The listing builds one solid part. Answer for the finished solid, in the listing's coordinates (mm). Face numbers are marked on the shaded views. A direction names the side the tool comes from. Coordinates: 2 decimals unless noted, no trailing zeros. Write each loop counter-clockwise with the first axis right and the second up, starting at its lowest first coordinate (ties: lowest second). Pieces come first, ordered by that corner, then holes.
(1) The part is cut by section A-A on x = 20. Determine the outline of the cut face in (y, z), plus the area to 3 significant figures.
(2) The part is cut by section C-C on y = 11. Determine the outline of the cut face in (x, z).
(3) Straight lines are drawn through the part: line 1 (Y direction, x = 20, z = 2.5); line 2 (X direction, y = 23.5, z = 14); line 3 (Z direction, x = 264, y = 31). For each, find the intervals that lie inside material, in ascending order.
(4) The part is cut by section B-B on z = 4.5. Determine the outline of the cut face in (x, y).
(5) Which of the six approach directions +Z, -Z, +X, -X, +Y, -Y give full straight-line access (tool end or side, diameter ignored) to the marked faces 1, 2 and 3?
(6) Given P1, Ø5, axis at y = 18.5, z = 14, coming from the -X side; P2, Ø20, axis at x = 19, y = 28.5, coming from the +Z side; P3, Ø11, axis at y = 14, z = 17.5, coming from the +X side, each flat-ended and moving along its own axis, determine where each tip first touches the part or whether it passes through.
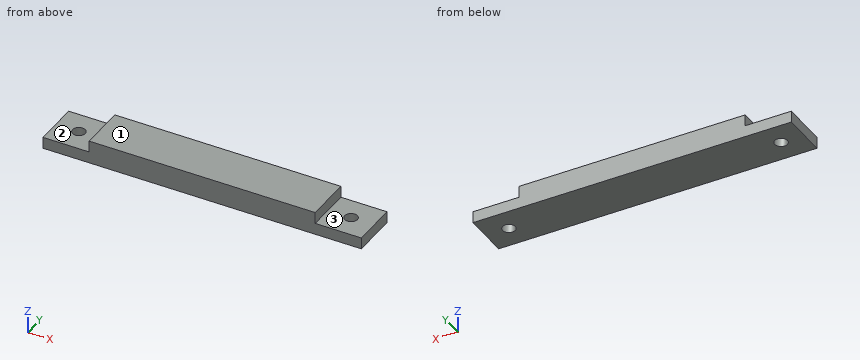
from build123d import *

# Parameters (mm, degrees)
ESQUISSE1_W        = 275.97
ESQUISSE1_H        = 40
ESQUISSE1_R        = 5.5
BOSS_EXTRU_1_DEPTH = 10
ESQUISSE2_W        = 195.97
ESQUISSE2_H        = 40
BOSS_EXTRU_2_DEPTH = 10


with BuildPart() as part:
    # Esquisse1 → Boss.-Extru.1 (new body)
    with BuildSketch(Plane.XY):
        with Locations((137.985, 20)):
            Rectangle(ESQUISSE1_W, ESQUISSE1_H)
        with Locations((20, 20)):
            Circle(ESQUISSE1_R, mode=Mode.SUBTRACT)
        with Locations(Location((255.97, 20, 0), (0, 0, 180))):
            Circle(ESQUISSE1_R, mode=Mode.SUBTRACT)
    extrude(amount=BOSS_EXTRU_1_DEPTH)

    # Esquisse2 → Boss.-Extru.2 (add)
    with BuildSketch(Plane.XY.offset(10)):
        with Locations((137.985, 20)):
            Rectangle(ESQUISSE2_W, ESQUISSE2_H)
    extrude(amount=BOSS_EXTRU_2_DEPTH)


solid = part.part
Model answer:
1. outline: (0, 0) - (14.5, 0) - (14.5, 10) - (0, 10) - close; (25.5, 0) - (40, 0) - (40, 10) - (25.5, 10) - close
1. area: 290 mm2
2. outline: (0, 0) - (275.97, 0) - (275.97, 10) - (235.97, 10) - (235.97, 20) - (40, 20) - (40, 10) - (0, 10) - close
3. line 1: y = 0 to 14.5, 25.5 to 40
3. line 2: x = 40 to 235.97
3. line 3: z = 0 to 10
4. outline: (0, 0) - (275.97, 0) - (275.97, 40) - (0, 40) - close; hole circle Ø11 at (20, 20); hole circle Ø11 at (255.97, 20)
5. face 1: +Z, +X, -X, +Y, -Y
5. face 2: +Z, -X, +Y, -Y
5. face 3: +Z, +X, +Y, -Y
6. P1: stops at x = 40
6. P2: stops at z = 10
6. P3: stops at x = 235.97
